Input: part model. Units: mm. Frame: model coordinates. Give positions to 0.01 mm unless a question says otherwise; leave off trailing zeros. Loops run counter-clockwise (first coordinate to the right, second up) from the corner with the lowest first, then second, coordinate; pieces in that order, holes last. Notation, with made-up numbers: (10, 47.5) -> (56, 47.5) arc R22 cw to (56, 79.5) -> close; hole circle Ø10 at (-15.5, -3). An arc over 180 degrees is marked (long way). Answer as a JSON object with one key per item and string values.
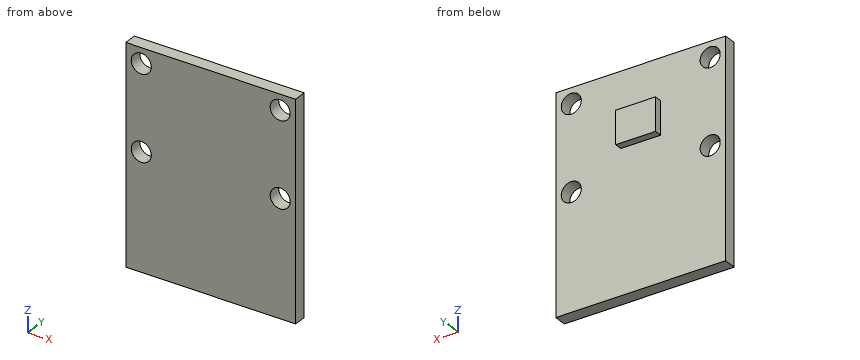
```python
from build123d import *

# Parameters (mm, degrees)
SKETCH1_W           = 22
SKETCH1_H           = 28
SKETCH1_R           = 1.3
BOSS_EXTRUDE1_DEPTH = 0.83
SKETCH2_W           = 5.16
SKETCH2_H           = 4.3
BOSS_EXTRUDE2_DEPTH = 1


with BuildPart() as part:
    # Sketch1 → Boss-Extrude1 (new, symmetric)
    with BuildSketch(Plane(origin=(0, 0, 0), x_dir=(1, 0, 0), z_dir=(0, 1, 0))):
        Rectangle(SKETCH1_W, SKETCH1_H)
        with Locations(Location((-9, -1, 0), (0, 0, 90))):
            Circle(SKETCH1_R, mode=Mode.SUBTRACT)
        with Locations(Location((9, -1, 0), (0, 0, 90))):
            Circle(SKETCH1_R, mode=Mode.SUBTRACT)
        with Locations(Location((-9, -12, 0), (0, 0, 90))):
            Circle(SKETCH1_R, mode=Mode.SUBTRACT)
        with Locations(Location((9, -12, 0), (0, 0, 90))):
            Circle(SKETCH1_R, mode=Mode.SUBTRACT)
    extrude(amount=BOSS_EXTRUDE1_DEPTH, both=True)

    # Sketch2 → Boss-Extrude2 (add)
    with BuildSketch(Plane(origin=(0, 0.83, 0), x_dir=(1, 0, 0), z_dir=(0, 1, 0))):
        with Locations((0, -6.5)):
            Rectangle(SKETCH2_W, SKETCH2_H)
    extrude(amount=BOSS_EXTRUDE2_DEPTH)


solid = part.part
```
Q1. Section B-B, the plane z = 12. Return the cut outline in (x, y).
Evaluation:
{"outline": "(-11, -0.83) -> (-10.3, -0.83) -> (-10.3, 0.83) -> (-11, 0.83) -> close; (-7.7, -0.83) -> (7.7, -0.83) -> (7.7, 0.83) -> (-7.7, 0.83) -> close; (10.3, -0.83) -> (11, -0.83) -> (11, 0.83) -> (10.3, 0.83) -> close"}
Q2. Section D-D, the plane y = 1.5. Return the cut outline in (x, z), then the cut area to 3 significant figures.
Evaluation:
{"outline": "(-2.58, 4.35) -> (2.58, 4.35) -> (2.58, 8.65) -> (-2.58, 8.65) -> close", "area": "22.2 mm2"}
Q3. Ray query, line 1 along X through (y, z) = (-0.2, 12); line 2 along Z through (x, y) = (-9, 0.2); line 3 along X through (y, z) = (-0.45, 2). Return the intervals inside material, ascending.
Evaluation:
{"line 1": "x = -11 to -10.3, -7.7 to 7.7, 10.3 to 11", "line 2": "z = -14 to -0.3, 2.3 to 10.7, 13.3 to 14", "line 3": "x = -11 to -9.83, -8.17 to 8.17, 9.83 to 11"}
Q4. Section A-A, the plane x = -9. Return the cut outline in (y, z).
Evaluation:
{"outline": "(-0.83, -14) -> (0.83, -14) -> (0.83, -0.3) -> (-0.83, -0.3) -> close; (-0.83, 2.3) -> (0.83, 2.3) -> (0.83, 10.7) -> (-0.83, 10.7) -> close; (-0.83, 13.3) -> (0.83, 13.3) -> (0.83, 14) -> (-0.83, 14) -> close"}
Q5. Section C-C, the plane y = -0.25. Return the cut outline in (x, z).
Evaluation:
{"outline": "(-11, -14) -> (11, -14) -> (11, 14) -> (-11, 14) -> close; hole circle Ø2.6 at (-9, 1); hole circle Ø2.6 at (-9, 12); hole circle Ø2.6 at (9, 1); hole circle Ø2.6 at (9, 12)"}
Q6. Pin query (flat end, axial travel): pin 1 (0.8 mm diameter, centred on x = 0.5, y = 1.5, fed in from -Z); pin 2 (0.5 mm diameter, centred on y = 1.5, z = 7, fed in from +X); pin 3 (5 mm diameter, centred on x = -4, z = -6, fed in from +Y); pin 4 (1.6 mm diameter, centred on x = -9, z = 12, fed in from +Y). Return the tip coordinate at first contact, or that it passes through.
Evaluation:
{"pin 1": "stops at z = 4.35", "pin 2": "stops at x = 2.58", "pin 3": "stops at y = 0.83", "pin 4": "passes through"}
